Geometry check sheet. Reference: the model listing, model coordinates, mm. Face numbers are marked on the shaded views. A direction names the side the tool comes from. Coordinates: 2 decimals unless noted, no trailing zeros. Write each loop counter-clockwise with the first axis right and the second up, starting at its lowest first coordinate (ties: lowest second). Pieces come first, ordered by that corner, then holes. Notation, with made-up numbers: (-6, 28.5) -> (3, 28.5) arc R13 cw to (3, 48.5) -> close; hole circle Ø9 at (22.25, 40.25). An arc over 180 degrees is marked (long way). Answer in a Markdown table with one row per item. Add a question column.
1. Cross-section at B-B on y = 8.5. Record the cut outline in (x, z).
2. Cross-section at D-D on y = 21.5. Record the cut outline in (x, z), and give its area (3 significant figures).
3. Depth check by flat-ended pin: P1, Ø6, axis at x = 4, z = -0.5, coming from the -Y side (3 decimals); P2, Ø5, axis at x = -4.5, y = 9, coming from the +Z side; P3, Ø0.5, axis at y = 19.5, z = -3, coming from the +X side; P4, Ø2.5, axis at x = -0.5, y = 28.5, coming from the -Z side. Enter the tip coordinate at first touch or a pass-through.
4. Scan lines: L1, parallel to Y at x = -3, z = 2.5 (3 decimals); L2, parallel to Y at x = 4, z = -1.25; L3, parallel to X at y = 16, z = 0. Record each from-to range of solid material in increasing order. Write a range as from..to.
5. Cross-section at A-A on z = 0. Record the cut outline in (x, y) (3 decimals), and give its area (3 significant figures).
6. Set-up check for the marked faces 1, 2 and 3: record each of +Z, -Z, +X, -X, +Y, -Y from which the full face is reachable in a straight line by a thin tool's end or side.
7. Cross-section at C-C on x = 1.5. Record the cut outline in (y, z) (3 decimals), and give its area (3 significant figures).
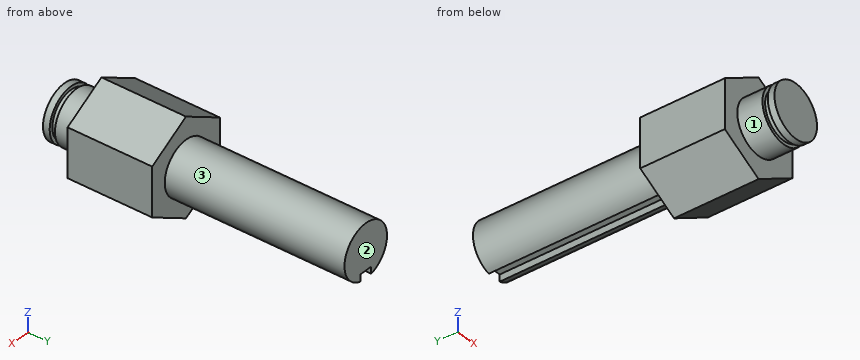
Autodesk Inventor part; units mm, degrees
ref_plane "YZ Plane" through (0, 0, 0) normal (1, 0, 0) x (0, 1, 0)
ref_plane "XZ Plane" through (0, 0, 0) normal (0, 1, 0) x (-1, 0, 0)
ref_plane "XY Plane" through (0, 0, 0) normal (0, 0, 1) x (1, 0, 0)
sketch "Sketch1" plane through (0, 0, 0) normal (0, 1, 0) x (-1, 0, 0)
  line L0 (0, -7.3323) -> (-6.35, -3.6662)
  line L1 (-6.35, -3.6662) -> (-6.35, 3.6662)
  line L2 (-6.35, 3.6662) -> (0, 7.3323)
  line L3 (0, 7.3323) -> (6.35, 3.6662)
  line L4 (6.35, 3.6662) -> (6.35, -3.6662)
  line L5 (6.35, -3.6662) -> (0, -7.3323)
  point P0 (0, 0)
  point P1 (0, 0)
  dimension "d0" = 12.7
extrude "Extrusion1" add sketch "Sketch1" along normal blind 12.7
sketch "Sketch2" plane through (0, 12.7, 0) normal (0, 1, 0) x (1, 0, 0)
  circle A0 centre (0, 0) radius 4
  dimension "d3" = 8
extrude "Extrusion2" add sketch "Sketch2" along normal blind 26.9926 and the other way blind 18.275
sketch "Sketch3" plane through (0, 39.6926, 0) normal (0, 1, 0) x (1, 0, 0)
  line L0 (-1.0287, 4) -> (1.0287, 4)
  line L1 (1.0287, 4) -> (1.0287, 2.8316)
  line L2 (1.0287, 2.8316) -> (-1.0287, 2.8316)
  line L3 (-1.0287, 2.8316) -> (-1.0287, 4)
  line L4 (0, 0) -> (0, 9.4373)
  circle A0 centre (0, 0) radius 4 construction
  circle A1 centre (0, 0) radius 4 construction
  dimension "d6" = 2.0574
  dimension "d8" = 1.1684
extrude "Extrusion3" cut sketch "Sketch3" against normal up to surface (26.9926 mm away)
sketch "Sketch4" plane through (0, 0, 0) normal (0, 0, 1) x (1, 0, 0)
  line L0 (4, -5.575) -> (4, 0)
  line L1 (4, -4.575) -> (3.5, -4.575)
  line L2 (3.5, -4.575) -> (3.5, -3.775)
  line L3 (3.5, -3.775) -> (4, -3.775)
  line L4 (4, -3.775) -> (4, -4.575)
  line L5 (0, -5.575) -> (0, 6.0324)
  line L6 (-4, -5.575) -> (4, -5.575)
  point P0 (0, 0)
  point P1 (4, -3.775)
  dimension "d13" = 0.8
  dimension "d14" = 7
  dimension "d16" = 1
revolve "Revolution1" cut sketch "Sketch4" angle 360 about axis through (0, -5.575, 0) along (0, 1, 0)
properties part number "Gear Shaft connector" material "Steel"
Results found:
| question | item | result |
|---|---|---|
| 1 | outline | (-6.35, -3.67) -> (0, -7.33) -> (6.35, -3.67) -> (6.35, 3.67) -> (0, 7.33) -> (-6.35, 3.67) -> close |
| 2 | outline | (-1.03, -3.87) -> (-1.03, -2.83) -> (1.03, -2.83) -> (1.03, -3.87) arc R4 ccw (long way) to start |
| 2 | area | 48.0 mm^2 |
| 3 | P1 | stops at y = -5.575 |
| 3 | P2 | stops at z = 6.18 |
| 3 | P3 | stops at x = 2.9 |
| 3 | P4 | stops at z = -3.87 |
| 4 | L1 | y = -5.575..-4.575, -3.775..39.693 |
| 4 | L2 | y = 0..12.7 |
| 4 | L3 | x = -4..4 |
| 5 | outline | (-6.35, 0) -> (-4, 0) -> (-4, -3.775) -> (-3.5, -3.775) -> (-3.5, -4.575) -> (-4, -4.575) -> (-4, -5.575) -> (4, -5.575) -> (4, -4.575) -> (3.5, -4.575) -> (3.5, -3.775) -> (4, -3.775) -> (4, 0) -> (6.35, 0) -> (6.35, 12.7) -> (4, 12.7) -> (4, 39.693) -> (-4, 39.693) -> (-4, 12.7) -> (-6.35, 12.7) -> close |
| 5 | area | 421 mm^2 |
| 6 | face 1 | -Y |
| 6 | face 2 | +Z, -Z, +X, -X, +Y |
| 6 | face 3 | +Y |
| 7 | outline | (-5.575, -3.708) -> (-4.575, -3.708) -> (-4.575, -3.162) -> (-3.775, -3.162) -> (-3.775, -3.708) -> (0, -3.708) -> (0, -6.466) -> (12.7, -6.466) -> (12.7, -3.708) -> (39.693, -3.708) -> (39.693, 3.708) -> (12.7, 3.708) -> (12.7, 6.466) -> (0, 6.466) -> (0, 3.708) -> (-3.775, 3.708) -> (-3.775, 3.162) -> (-4.575, 3.162) -> (-4.575, 3.708) -> (-5.575, 3.708) -> close |
| 7 | area | 405 mm^2 |
